```python
from build123d import *

# Parameters (mm, degrees)
CROQUIS1_R              = 24.5
SALIENTE_EXTRUIR1_DEPTH = 4
CROQUIS2_R              = 2
CORTAR_EXTRUIR1_DEPTH   = 35.878360053
MATRIZC1_COUNT          = 6
SALIENTE_EXTRUIR2_START = 5
CROQUIS3_R              = 47.5
CROQUIS3_R_2            = 2
SALIENTE_EXTRUIR2_DEPTH = 5
CROQUIS6_R              = 1.5
CORTAR_EXTRUIR2_DEPTH   = 68.775364256
CORTAR_EXTRUIR3_START   = -4
CROQUIS7_R              = 3.5
CROQUIS7_R_2            = 1.5
CORTAR_EXTRUIR3_DEPTH   = 4


with BuildPart() as part:
    # Croquis1 → Saliente-Extruir1 (new body)
    with BuildSketch(Plane(origin=(0, 0, 0), x_dir=(1, 0, 0), z_dir=(0, 1, 0))):
        with Locations(Location((0, 0, 0), (0, 0, 270))):
            Circle(CROQUIS1_R)
    extrude(amount=SALIENTE_EXTRUIR1_DEPTH)

    # Croquis2 → Cortar-Extruir1 (cut, through all)
    with BuildSketch(Plane(origin=(0, 4, 0), x_dir=(1, 0, 0), z_dir=(0, 1, 0))):
        with Locations(Location((0, 16, 0), (0, 0, 270))):
            Circle(CROQUIS2_R)
    cortar_extruir1 = extrude(amount=-CORTAR_EXTRUIR1_DEPTH, mode=Mode.SUBTRACT)

    # MatrizC1: Cortar-Extruir1 ×6 about axis
    matrizc1_axis = Axis((0, 0, 0), (0, 1, 0))
    for i in range(1, MATRIZC1_COUNT):
        add(cortar_extruir1.rotate(matrizc1_axis, i * 360 / MATRIZC1_COUNT), mode=Mode.SUBTRACT)

    # Croquis3 → Saliente-Extruir2 (add)
    with BuildSketch(Plane(origin=(0, 4, 0), x_dir=(1, 0, 0), z_dir=(0, 1, 0)).offset(SALIENTE_EXTRUIR2_START)):
        with Locations(Location((0, 0, 0), (0, 0, 270))):
            Circle(CROQUIS3_R)
        with Locations(Location((13.856406461, 8, 0), (0, 0, 270))):
            Circle(CROQUIS3_R_2, mode=Mode.SUBTRACT)
        with Locations(Location((13.856406461, -8, 0), (0, 0, 270))):
            Circle(CROQUIS3_R_2, mode=Mode.SUBTRACT)
        with Locations(Location((0, -16, 0), (0, 0, 270))):
            Circle(CROQUIS3_R_2, mode=Mode.SUBTRACT)
        with Locations(Location((-13.856406461, -8, 0), (0, 0, 270))):
            Circle(CROQUIS3_R_2, mode=Mode.SUBTRACT)
        with Locations(Location((-13.856406461, 8, 0), (0, 0, 270))):
            Circle(CROQUIS3_R_2, mode=Mode.SUBTRACT)
        with Locations(Location((0, 16, 0), (0, 0, 270))):
            Circle(CROQUIS3_R_2, mode=Mode.SUBTRACT)
    extrude(amount=-SALIENTE_EXTRUIR2_DEPTH)

    # Croquis6 → Cortar-Extruir2 (cut, through all)
    with BuildSketch(Plane(origin=(0, 9, 0), x_dir=(1, 0, 0), z_dir=(0, 1, 0))):
        with Locations(Location((-35, 15, 0), (0, 0, 270))):
            Circle(CROQUIS6_R)
        with Locations(Location((-35, 0, 0), (0, 0, 270))):
            Circle(CROQUIS6_R)
        with Locations(Location((-35, -15, 0), (0, 0, 270))):
            Circle(CROQUIS6_R)
    cortar_extruir2 = extrude(amount=-CORTAR_EXTRUIR2_DEPTH, mode=Mode.SUBTRACT)

    # Simetría1: Cortar-Extruir2 across plane
    add(cortar_extruir2.mirror(Plane(origin=(0, 0, 0), x_dir=(0, 0, 1), z_dir=(1, 0, 0))), mode=Mode.SUBTRACT)

    # Croquis7 → Cortar-Extruir3 (cut)
    # profile 1 of 6: a face of its own
    with BuildSketch(Plane.XZ.offset(-4).offset(CORTAR_EXTRUIR3_START)):
        with Locations(Location((35, 15, 0), (0, 0, 270))):
            Circle(CROQUIS7_R)
        with Locations(Location((35, 15, 0), (0, 0, 90))):
            Circle(CROQUIS7_R_2, mode=Mode.SUBTRACT)
    # profile 2 of 6: a face of its own
    with BuildSketch(Plane.XZ.offset(-4).offset(CORTAR_EXTRUIR3_START)):
        with Locations(Location((35, 0, 0), (0, 0, 270))):
            Circle(CROQUIS7_R)
        with Locations(Location((35, 0, 0), (0, 0, 90))):
            Circle(CROQUIS7_R_2, mode=Mode.SUBTRACT)
    # profile 3 of 6: a face of its own
    with BuildSketch(Plane.XZ.offset(-4).offset(CORTAR_EXTRUIR3_START)):
        with Locations(Location((35, -15, 0), (0, 0, 270))):
            Circle(CROQUIS7_R)
        with Locations(Location((35, -15, 0), (0, 0, 90))):
            Circle(CROQUIS7_R_2, mode=Mode.SUBTRACT)
    # profile 4 of 6: a face of its own
    with BuildSketch(Plane.XZ.offset(-4).offset(CORTAR_EXTRUIR3_START)):
        with Locations(Location((-35, 15, 0), (0, 0, 270))):
            Circle(CROQUIS7_R)
        with Locations(Location((-35, 15, 0), (0, 0, 90))):
            Circle(CROQUIS7_R_2, mode=Mode.SUBTRACT)
    # profile 5 of 6: a face of its own
    with BuildSketch(Plane.XZ.offset(-4).offset(CORTAR_EXTRUIR3_START)):
        with Locations(Location((-35, 0, 0), (0, 0, 270))):
            Circle(CROQUIS7_R)
        with Locations(Location((-35, 0, 0), (0, 0, 90))):
            Circle(CROQUIS7_R_2, mode=Mode.SUBTRACT)
    # profile 6 of 6: a face of its own
    with BuildSketch(Plane.XZ.offset(-4).offset(CORTAR_EXTRUIR3_START)):
        with Locations(Location((-35, -15, 0), (0, 0, 270))):
            Circle(CROQUIS7_R)
        with Locations(Location((-35, -15, 0), (0, 0, 90))):
            Circle(CROQUIS7_R_2, mode=Mode.SUBTRACT)
    extrude(amount=CORTAR_EXTRUIR3_DEPTH, mode=Mode.SUBTRACT)


solid = part.part
```
Verification items for the finished model (mm, model axes). A direction names the side the tool comes from. Round coordinates to 2 decimals unless told otherwise and drop trailing zeros. Write each loop counter-clockwise with the first axis right and the second up, starting at its lowest first coordinate (ties: lowest second). Pieces come first, ordered by that corner, then holes. Notation, with made-up numbers: (36, 41) - (64, 41) arc R20 cw to (64, 58) - close; hole circle Ø10 at (57, 41.5). An arc over 180 degrees is marked (long way). Answer as a JSON object with one key per item and string values. Group by question number.
Q1. Go/stop test with flat-tipped pins: pin 1 Ø4 at (x, y) = (-11, 4.5) entering from -Z; pin 2 Ø5 at (x, z) = (-19.5, 28.5) entering from -Y; pin 3 Ø2 at (x, z) = (36, 15) entering from -Y. Record where each tip stops, or that it passes through.
Q2. Thickness scan on line 1 (X direction, y = 4.9, z = 15); line 2 (X direction, y = 3.15, z = -8); line 3 (Z direction, x = 35, y = 8.4). Record the ranges inside material, lowest first.
Q3. Section check C-C, the plane y = 2. Enter the section's corners in (x, z), plus the area to 3 significant figures.
Q4. Mould release check, pull along X, two halves, no side actions. Record for faces 3 (the cylindrical face through (2, 5, 16)), 4 (the cylindrical face through (-46.37, 6.54, -10.3)), 5 (the flat face through (-20, 4, 20)): released by +X, released by -X, zero draft, split by the parting line, or undercut.
Q5. Section check B-B, the plane y = 6.75. Give the number of separate pieces and of enclosed holes in the cut face, plus the area to 3 significant figures.
Q6. Tool access check on faces 1 (the cylindrical face through (38.47, 6.03, -14.54)), 2 (the cylindrical face through (-35.9, 8.5, 13.8)). Record the directions out of +Z, -Z, +X, -X, +Y, -Y that give a thin tool (end or side, any length) a straight path to the whole face; none if there is none.
Q7. Section check D-D, the plane x = 35. Enter the section's corners in (y, z), plus the area to 3 significant figures.
Q8. Section check A-A, the plane x = 0. Enter the section's corners in (y, z), plus the area to 3 significant figures.
Found:
{
 "1": {"pin 1": "stops at z = -46.64", "pin 2": "stops at y = 4", "pin 3": "stops at y = 8"},
 "2": {"line 1": "x = -45.07 to -38.5, -31.5 to -1.73, 1.73 to 31.5, 38.5 to 45.07", "line 2": "x = -23.16 to -15.86, -11.86 to 11.86, 15.86 to 23.16", "line 3": "z = -32.11 to -16.5, -13.5 to -1.5, 1.5 to 13.5, 16.5 to 32.11"},
 "3": {"outline": "circle Ø49 at (0, 0); hole circle Ø4 at (-13.86, -8); hole circle Ø4 at (-13.86, 8); hole circle Ø4 at (0, -16); hole circle Ø4 at (0, 16); hole circle Ø4 at (13.86, -8); hole circle Ø4 at (13.86, 8)", "area": "1,810 mm^2"},
 "4": {"face 3": "undercut", "face 4": "split by the parting line", "face 5": "zero draft"},
 "5": {"separate pieces": "1", "enclosed holes": "12", "area": "6,780 mm^2"},
 "6": {"face 1": "-Y", "face 2": "+Y, -Y"},
 "7": {"outline": "(4, -32.11) - (9, -32.11) - (9, -16.5) - (8, -16.5) - (8, -18.5) - (4, -18.5) - close; (4, -11.5) - (8, -11.5) - (8, -13.5) - (9, -13.5) - (9, -1.5) - (8, -1.5) - (8, -3.5) - (4, -3.5) - close; (4, 3.5) - (8, 3.5) - (8, 1.5) - (9, 1.5) - (9, 13.5) - (8, 13.5) - (8, 11.5) - (4, 11.5) - close; (4, 18.5) - (8, 18.5) - (8, 16.5) - (9, 16.5) - (9, 32.11) - (4, 32.11) - close", "area": "228 mm^2"},
 "8": {"outline": "(0, -24.5) - (4, -24.5) - (4, -47.5) - (9, -47.5) - (9, -18) - (0, -18) - close; (0, -14) - (9, -14) - (9, 14) - (0, 14) - close; (0, 18) - (9, 18) - (9, 47.5) - (4, 47.5) - (4, 24.5) - (0, 24.5) - close", "area": "599 mm^2"}
}
